```python
from build123d import *

# Parameters (mm, degrees)
SKETCH1_W           = 152.4
SKETCH1_H           = 152.4
SKETCH1_R           = 5
SKETCH1_R_2         = 12.7
BOSS_EXTRUDE1_DEPTH = 3


with BuildPart() as part:
    # Sketch1 → Boss-Extrude1 (new body)
    # profile 1 of 5: a face of its own
    with BuildSketch(Plane(origin=(0, 0, 0), x_dir=(1, 0, 0), z_dir=(0, 1, 0))):
        Rectangle(SKETCH1_W, SKETCH1_H)
        with Locations((57.513684792, -57.513684792)):
            Circle(SKETCH1_R, mode=Mode.SUBTRACT)
        with Locations((57.513684792, 57.513684792)):
            Circle(SKETCH1_R, mode=Mode.SUBTRACT)
        with Locations((-57.513684792, 57.513684792)):
            Circle(SKETCH1_R, mode=Mode.SUBTRACT)
        with Locations((-57.513684792, -57.513684792)):
            Circle(SKETCH1_R, mode=Mode.SUBTRACT)
        with Locations(Location((-25.4, 0, 0), (0, 0, 270))):
            Circle(SKETCH1_R_2, mode=Mode.SUBTRACT)
    # profile 2 of 5: a face of its own
    with BuildSketch(Plane(origin=(0, 0, 0), x_dir=(1, 0, 0), z_dir=(0, 1, 0))):
        with Locations((57.513684792, -57.513684792)):
            Circle(SKETCH1_R)
    # profile 3 of 5: a face of its own
    with BuildSketch(Plane(origin=(0, 0, 0), x_dir=(1, 0, 0), z_dir=(0, 1, 0))):
        with Locations((-57.513684792, -57.513684792)):
            Circle(SKETCH1_R)
    # profile 4 of 5: a face of its own
    with BuildSketch(Plane(origin=(0, 0, 0), x_dir=(1, 0, 0), z_dir=(0, 1, 0))):
        with Locations((57.513684792, 57.513684792)):
            Circle(SKETCH1_R)
    # profile 5 of 5: a face of its own
    with BuildSketch(Plane(origin=(0, 0, 0), x_dir=(1, 0, 0), z_dir=(0, 1, 0))):
        with Locations((-57.513684792, 57.513684792)):
            Circle(SKETCH1_R)
    extrude(amount=-BOSS_EXTRUDE1_DEPTH)


solid = part.part
```
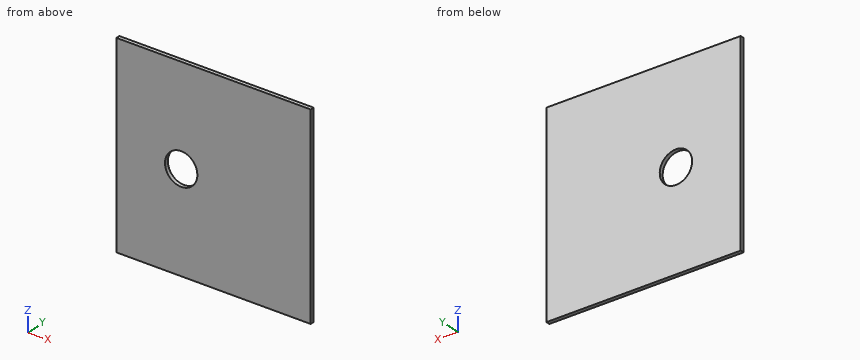
Geometry: final body of the model. Coordinates: model frame, mm. Coordinates: 2 decimals unless noted, no trailing zeros. Order: outer loops, then holes, each group sorted by start corner. A loop starts at its lowest first (then second) coordinate and runs counter-clockwise, first axis right, second up. Notation, with made-up numbers: M -24.5,25 L 32.5,25 A32 ccw 32.5,56 Z; hole C 54,65.5 d4. An arc over 180 degrees is marked long. Answer in a Markdown table with one row per item. Add a question column.
Q1. Section query C-C on y = -1.75. Return the cut outline in (x, z).
Q2. Line query: L1, parallel to X at y = -1, z = 0; L2, parallel to X at y = -1.75, z = 2.5. Output: solid intervals per line, ascending.
Q3. Section query B-B on x = -25.4. Return the cut outline in (y, z).
Q4. Section query A-A on z = 0. Return the cut outline in (x, y), and give its area (3 significant figures).
Completed:
| question | item | result |
|---|---|---|
| 1 | outline | M -76.2,-76.2 L 76.2,-76.2 L 76.2,76.2 L -76.2,76.2 Z; hole C -25.4,0 d25.4 |
| 2 | L1 | x = -76.2 to -38.1, -12.7 to 76.2 |
| 2 | L2 | x = -76.2 to -37.85, -12.95 to 76.2 |
| 3 | outline | M -3,-76.2 L 0,-76.2 L 0,-12.7 L -3,-12.7 Z; M -3,12.7 L 0,12.7 L 0,76.2 L -3,76.2 Z |
| 4 | outline | M -76.2,-3 L -38.1,-3 L -38.1,0 L -76.2,0 Z; M -12.7,-3 L 76.2,-3 L 76.2,0 L -12.7,0 Z |
| 4 | area | 381 mm2 |
